Verification items for the finished model (mm, model axes). A direction names the side the tool comes from. Coordinates: 2 decimals unless noted, no trailing zeros. Order: outer loops, then holes, each group sorted by start corner. A loop starts at its lowest first (then second) coordinate and runs counter-clockwise, first axis right, second up. Notation, with made-up numbers: (58.25, 60) -> (66.25, 60) arc R24 cw to (66.25, 98) -> close; hole circle Ø5 at (-8.75, 78.25). An arc over 180 degrees is marked (long way). Write each question's results on one line, items separated by ' | '. Start each with the question number.
(1) Cross-section at D-D on y = 21.5. Enter the section's corners in (x, z), and give its area (3 significant figures).
(2) Cross-section at B-B on x = 8. Enter the section's corners in (y, z).
(3) Draft check along Y on faces 4 (the flat face through (15, 24, 0)), 5 (the flat face through (17, 14, 0)), 6 (the flat face through (-1, 10, -5)). Enter one of: +Y half, -Y half, draft (parallel to the pull), parting line (faces both ways), or undercut.
(4) Set-up check for faces 1 (the flat face through (0, 31, 0)), 2 (the flat face through (15, 17, 0)), 3 (the flat face through (18, 5, 0)): record each of +Z, -Z, +X, -X, +Y, -Y from which the full face is reachable in a straight line by a thin tool's end or side.
(5) Cross-section at C-C on z = -3. Enter the section's corners in (x, y), and give its area (3 significant figures).
(6) Thickness scan on probe 1 along Y at (x, z) = (4, 2); probe 2 along Z at (x, y) = (-7, 9.5); probe 3 along X at (y, z) = (14.5, 4.25). Record the ranges inside material, lowest first. Write a range as [from, to].
(7) Go/stop test with flat-tipped pins: pin 1 (0.8 mm diameter, centred on x = -7.5, z = 6, fed in from -Y); pin 2 (4 mm diameter, centred on y = 8, z = 2, fed in from +X); pin 3 (3 mm diameter, centred on x = -6.5, z = 0, fed in from +Y); pin 4 (2.5 mm diameter, centred on y = 9.5, z = 0, fed in from +X). Record where each tip stops, or that it passes through.
(8) Cross-section at A-A on y = 9.5. Enter the section's corners in (x, z), and give its area (3 significant figures).
```python
from build123d import *

# Parameters (mm, degrees)
BOSS_EXTRUDE1_DEPTH = 5
SKETCH2_R           = 2.1
CUT_EXTRUDE1_DEPTH  = 10
SKETCH3_R           = 10
BOSS_EXTRUDE2_DEPTH = 1
SKETCH4_R           = 2.75
BOSS_EXTRUDE3_DEPTH = 5
SKETCH5_W           = 50
SKETCH5_H           = 30
SKETCH5_W_2         = 34
SKETCH5_H_2         = 14
CUT_EXTRUDE2_DEPTH  = 52.14684741
CUT_EXTRUDE3_START  = -1
CUT_EXTRUDE3_DEPTH  = 1
CUT_EXTRUDE4_START  = -1
CUT_EXTRUDE4_DEPTH  = 1
CHAMFER1_SIZE       = 3
CHAMFER2_SIZE       = 3
BOSS_EXTRUDE4_DEPTH = 1
BOSS_EXTRUDE5_START = 1
BOSS_EXTRUDE5_DEPTH = 1


with BuildPart() as part:
    # Sketch1 → Boss-Extrude1 (new, symmetric)
    with BuildSketch(Plane.XY):
        Polygon((15, 5), (15, 0), (0, 0), (0, 19), (15, 19), (15, 14), (20, 14), (20, 24), (-10, 24), (-10, -5), (20, -5), (20, 5), align=None)
    extrude(amount=BOSS_EXTRUDE1_DEPTH, both=True)

    # Sketch2 → Cut-Extrude1 (cut)
    with BuildSketch(Plane.ZY.offset(10)):
        with Locations(Location((0, 9.5, 0), (0, 0, 270))):
            Circle(SKETCH2_R)
    extrude(amount=-CUT_EXTRUDE1_DEPTH, mode=Mode.SUBTRACT)

    # Sketch3 → Boss-Extrude2 (add)
    with BuildSketch(Plane(origin=(0, 24, 0), x_dir=(1, 0, 0), z_dir=(0, 1, 0))):
        with Locations(Location((0, 0, 0), (0, 0, 180))):
            Circle(SKETCH3_R)
    extrude(amount=BOSS_EXTRUDE2_DEPTH)

    # Sketch4 → Boss-Extrude3 (add)
    with BuildSketch(Plane(origin=(0, 0, 0), x_dir=(0.866025403784438, 0, -0.500000000000001), z_dir=(0.500000000000001, 0, 0.866025403784438))):
        with BuildLine():
            Line((10, 25), (-10, 25))
            Line((-10, 25), (-4.615384615, 37.923076923))
            ThreePointArc((-4.615384615, 37.923076923), (0, 41), (4.615384615, 37.923076923))
            Line((4.615384615, 37.923076923), (10, 25))
        make_face()
        with Locations((0, 36)):
            Circle(SKETCH4_R, mode=Mode.SUBTRACT)
    extrude(amount=BOSS_EXTRUDE3_DEPTH)

    # Sketch5 → Cut-Extrude2 (cut, through all)
    with BuildSketch(Plane.XZ.offset(5)):
        with Locations((5, 0)):
            Rectangle(SKETCH5_W, SKETCH5_H)
        with Locations((5, 0)):
            Rectangle(SKETCH5_W_2, SKETCH5_H_2, mode=Mode.SUBTRACT)
    extrude(amount=-CUT_EXTRUDE2_DEPTH, mode=Mode.SUBTRACT)

    # Sketch6 → Cut-Extrude3 (cut)
    with BuildSketch(Plane(origin=(0, 25, 0), x_dir=(1, 0, 0), z_dir=(0, 1, 0)).offset(CUT_EXTRUDE3_START)):
        with BuildLine():
            Line((7.141428429, 7), (-7.141428429, 7))
            ThreePointArc((-7.141428429, 7), (-9.920851384, 1.255670262), (-8.660254038, -5))
            Line((-8.660254038, -5), (8.660254038, 5))
            ThreePointArc((8.660254038, 5), (7.963874195, 6.047868038), (7.141428429, 7))
        make_face()
    extrude(amount=CUT_EXTRUDE3_DEPTH, mode=Mode.SUBTRACT)

    # Sketch7 → Cut-Extrude4 (cut)
    with BuildSketch(Plane(origin=(0, 25, 0), x_dir=(1, 0, 0), z_dir=(0, 1, 0)).offset(CUT_EXTRUDE4_START)):
        with BuildLine():
            Line((-2.124355653, -7), (7.141428429, -7))
            ThreePointArc((7.141428429, -7), (9.257815193, -3.780589618), (10, 0))
            Line((10, 0), (-2.124355653, -7))
        make_face()
    extrude(amount=CUT_EXTRUDE4_DEPTH, mode=Mode.SUBTRACT)

    # Chamfer1
    chamfer1_edges = [part.edges().sort_by_distance(p)[0] for p in [
        (5.669872981, 24, 2.5),
    ]]
    chamfer(chamfer1_edges, length=CHAMFER1_SIZE)

    # Chamfer2
    # the kernel refuses this chamfer: 3 mm, written as the material it adds along each edge
    with BuildSketch(Plane(origin=(9.054794926, 24, 5), x_dir=(0, -0.9996219169112968, -0.02749587661058648), z_dir=(-1, 0, 0))) as chamfer2_piece_1_section:
        Polygon((CHAMFER2_SIZE * 0.999621916911, CHAMFER2_SIZE * 0.0274958766106), (-CHAMFER2_SIZE * 0.0274958766106, CHAMFER2_SIZE * 0.999621916911), (0, 0), align=None)
    chamfer2_piece_1 = extrude(amount=25.430097928, mode=Mode.PRIVATE)
    chamfer2_piece_1 = split(chamfer2_piece_1, bisect_by=Plane(origin=(-3.023607394, 22.869371877, 7.519183235), z_dir=(-0.5000000000000006, 0, -0.8660254037844384)), keep=Keep.TOP, mode=Mode.PRIVATE)
    chamfer2_piece_1 = chamfer2_piece_1 & Plane(origin=(0, 22.869371877, 0), x_dir=(-1, 0, 0), z_dir=(0, -1, 0)) * Cylinder(10, 63, mode=Mode.PRIVATE)
    chamfer2_piece_1 = split(chamfer2_piece_1, bisect_by=Plane(origin=(-4.051544608, 22.869371877, 7), z_dir=(0, 0, -1)), keep=Keep.TOP, mode=Mode.PRIVATE)
    add(chamfer2_piece_1)

    # Sketch9 → Boss-Extrude4 (add)
    with BuildSketch(Plane(origin=(0, 24, 0), x_dir=(1, 0, 0), z_dir=(0, 1, 0))):
        Polygon((8.660254038, 5), (-10, 5), (-10, -5), (-8.660254038, -5), align=None)
    extrude(amount=BOSS_EXTRUDE4_DEPTH)

    # Sketch10 → Boss-Extrude5 (add)
    with BuildSketch(Plane.XZ.offset(-25).offset(BOSS_EXTRUDE5_START)):
        with BuildLine():
            Line((8.660254038, -5), (12.160254038, 1.062177826))
            Line((12.160254038, 1.062177826), (9.684658438, 2.491463612))
            ThreePointArc((9.684658438, 2.491463612), (9.907797949, -1.354820946), (8.660254038, -5))
        make_face()
    extrude(amount=-BOSS_EXTRUDE5_DEPTH)


solid = part.part
```
Results are:
1) outline: (-10, -5) -> (20, -5) -> (20, 5) -> (1.34, 5) -> (0.47, 5.5) -> (-8.35, 5.5) arc R10 ccw to (-8.66, 5) -> (-10, 5) -> close | area: 305 mm2
2) outline: (-5, -5) -> (0, -5) -> (0, 5) -> (-5, 5) -> close; (19, -5) -> (25, -5) -> (25, -4.62) -> (26.83, -4.62) -> (33.76, 1.15) -> (27, 1.15) -> (24, 4.62) -> (24, 5) -> (19, 5) -> close
3) face 4: +Y half | face 5: undercut | face 6: draft
4) face 1: -Z, -X, +Y | face 2: +Z, -Z | face 3: +Z, -Z, +X
5) outline: (-10, -5) -> (20, -5) -> (20, 5) -> (15, 5) -> (15, 0) -> (0, 0) -> (0, 19) -> (15, 19) -> (15, 14) -> (20, 14) -> (20, 24) -> (9.81, 24) -> (9.81, 25) -> (5.2, 34.6) -> (5.2, 25) -> (-10, 25) -> close | area: 582 mm2
6) probe 1: y = [-5, 0], [19, 34.78], [37.22, 40.35] | probe 2: z = [-5, -2.1], [2.1, 5] | probe 3: x = [-10, 0], [15, 20]
7) pin 1: stops at y = 21.6 | pin 2: stops at x = 0 | pin 3: stops at y = 25 | pin 4: passes through
8) outline: (-10, -5) -> (0, -5) -> (0, -2.1) -> (-10, -2.1) -> close; (-10, 2.1) -> (0, 2.1) -> (0, 5) -> (-10, 5) -> close | area: 58.0 mm2
